```python
from build123d import *

# Parameters (mm, degrees)
SKETCH2_R           = 5
SKETCH2_R_2         = 2
SKETCH2_R_3         = 1.5
BOSS_EXTRUDE1_DEPTH = 5
SKETCH3_R           = 4.5
CUT_EXTRUDE1_DEPTH  = 3.5
BOSS_EXTRUDE2_START = -5
SKETCH4_R           = 5
SKETCH4_R_2         = 3.5
BOSS_EXTRUDE2_DEPTH = 1


with BuildPart() as part:
    # Sketch2 → Boss-Extrude1 (new body)
    with BuildSketch(Plane(origin=(0, 0, 0), x_dir=(0, 0, -1), z_dir=(1, 0, 0))):
        with BuildLine():
            Line((58.308676511, 0), (-58.308676511, 0))
            Line((-58.308676511, 0), (-75.243665272, -8.783179062))
            ThreePointArc((-75.243665272, -8.783179062), (-87.141316573, -21.040619401), (-89.217284989, -37.996128985))
            ThreePointArc((-89.217284989, -37.996128985), (-73.76298075, -50.59971931), (-58.308676511, -37.996128985))
            Line((-58.308676511, -37.996128985), (-7, -37.996128985))
            Line((-7, -37.996128985), (-2.757359313, -42.238769672))
            ThreePointArc((-2.757359313, -42.238769672), (0, -43.380905296), (2.757359313, -42.238769672))
            Line((2.757359313, -42.238769672), (7, -37.996128985))
            Line((7, -37.996128985), (58.308676511, -37.996128985))
            ThreePointArc((58.308676511, -37.996128985), (87.163327852, -44.335147902), (90.85122644, -15.023486932))
            Line((90.85122644, -15.023486932), (58.308676511, 0))
        make_face()
        with Locations((-74.370815413, -37.996128985)):
            Circle(SKETCH2_R, mode=Mode.SUBTRACT)
        with Locations((75.629184587, -37.996128985)):
            Circle(SKETCH2_R_2, mode=Mode.SUBTRACT)
        with Locations((0, -38)):
            Circle(SKETCH2_R_3, mode=Mode.SUBTRACT)
        with BuildLine():
            Line((-58.308676511, -27), (58.308676511, -27))
            ThreePointArc((58.308676511, -27), (61.808676511, -23.5), (58.308676511, -20))
            Line((58.308676511, -20), (-58.308676511, -20))
            ThreePointArc((-58.308676511, -20), (-61.808676511, -23.5), (-58.308676511, -27))
        make_face(mode=Mode.SUBTRACT)
    extrude(amount=BOSS_EXTRUDE1_DEPTH)

    # Sketch3 → Cut-Extrude1 (cut)
    with BuildSketch(Plane(origin=(5, 0, 0), x_dir=(0, 0, -1), z_dir=(1, 0, 0))):
        with Locations((75.629184587, -37.996128985)):
            Circle(SKETCH3_R)
    extrude(amount=-CUT_EXTRUDE1_DEPTH, mode=Mode.SUBTRACT)

    # Sketch4 → Boss-Extrude2 (add)
    with BuildSketch(Plane(origin=(5, 0, 0), x_dir=(0, 0, -1), z_dir=(1, 0, 0)).offset(BOSS_EXTRUDE2_START)):
        with Locations((-74.370815413, -37.996128985)):
            Circle(SKETCH4_R)
        with Locations((-74.370815413, -37.996128985)):
            Circle(SKETCH4_R_2, mode=Mode.SUBTRACT)
    extrude(amount=BOSS_EXTRUDE2_DEPTH)


solid = part.part
```
Geometry check sheet. Reference: the model listing, model coordinates, mm. A direction names the side the tool comes from. Round coordinates to 2 decimals unless told otherwise and drop trailing zeros. Write each loop counter-clockwise with the first axis right and the second up, starting at its lowest first coordinate (ties: lowest second). Pieces come first, ordered by that corner, then holes. Notation, with made-up numbers: (83.5, 85) - (138.5, 85) arc R7 cw to (138.5, 93) - close; hole circle Ø5 at (82.25, 89.5). An arc over 180 degrees is marked (long way). Write each question's results on one line, items separated by ' | '.
(1) Sectioned sample at B-B, the plane x = 3.1. Enter the section's corners in (y, z), plus the area to 3 significant figures.
Computed:
outline: (-42.24, -2.76) - (-38, -7) - (-38, -58.31) arc R20 ccw (long way) to (-15.02, -90.85) - (0, -58.31) - (0, 58.31) - (-8.78, 75.24) arc R26.8 ccw to (-38, 89.22) arc R15.78 ccw to (-38, 58.31) - (-38, 7) - (-42.24, 2.76) arc R3.9 ccw to start; hole circle Ø10 at (-38, 74.37); hole circle Ø9 at (-38, -75.63); hole circle Ø3 at (-38, 0); hole (-27, -58.31) arc R3.5 ccw to (-20, -58.31) - (-20, 58.31) arc R3.5 ccw to (-27, 58.31) - close | area: 5,980 mm^2
(2) Sectioned sample at C-C, the plane y = -46. Enter the section's corners in (x, z).
Computed:
outline: (0, -84.34) - (5, -84.34) - (5, -66.92) - (0, -66.92) - close; (0, 62.63) - (5, 62.63) - (5, 84.9) - (0, 84.9) - close
(3) Draft check along Z on faces 1 (the face through (5, -19, -2)), 2 (the face through (2.465, -20.822, 87.035)), 3 (the face through (2.97, -39.91, 69.75)). Enter one of: pulls with the +Z half, pulls with the -Z half, needs draft (parallel to the pull), parting line crosses it, or undercut.
Computed:
face 1: needs draft | face 2: pulls with the +Z half | face 3: undercut
(4) Thickness scan on probe 1 along Y at (x, z) = (1.1, -16.5); probe 2 along Z at (x, y) = (4.65, -40.5); probe 3 along Z at (x, y) = (0.9, -37.5). Record the ranges inside material, lowest first. Write a range as from..to.
Computed:
probe 1: y = -38..-27, -20..0 | probe 2: z = -91.24..-79.37, -71.89..-60.02, -4.5..4.5, 59.04..70.04, 78.7..88.48 | probe 3: z = -93.23..-77.57, -73.69..-1.41, 1.41..70.91, 77.84..89.31
(5) Set-up check for faces 4 (the face through (2.46, -4.33, 66.66)), 5 (the face through (2, -37.996, -32)), 6 (the face through (2.465, -23.577, -61.808)), 7 (the face through (1.5, -40, -77)): record each of +Z, -Z, +X, -X, +Y, -Y from which the full face is reachable in a straight line by a thin tool's end or side.
Computed:
face 4: +Z, +X, -X, +Y | face 5: +X, -X, -Y | face 6: +X, -X | face 7: +X
(6) Sectioned sample at D-D, the plane y = -6.5. Enter the section's corners in (x, z), plus the area to 3 significant figures.
Computed:
outline: (0, -72.39) - (5, -72.39) - (5, 70.84) - (0, 70.84) - close | area: 716 mm^2
(7) Sectioned sample at A-A, the plane z = -18.5. Enter the section's corners in (x, y), plus the area to 3 significant figures.
Computed:
outline: (0, -38) - (5, -38) - (5, -27) - (0, -27) - close; (0, -20) - (5, -20) - (5, 0) - (0, 0) - close | area: 155 mm^2
(8) Depth check by flat-ended pin: pin 1 Ø1.5 at (x, z) = (2, 11) entering from +Y; pin 2 Ø4.5 at (y, z) = (-38, -75.63) entering from +X; pin 3 Ø5 at (y, z) = (-37, 75.5) entering from +X; pin 4 Ø3 at (x, z) = (2, -5) entering from -Y. Enter the tip coordinate at first touch or a pass-through.
Computed:
pin 1: stops at y = 0 | pin 2: stops at x = 1.5 | pin 3: stops at x = 1 | pin 4: stops at y = -41.5
